The listing builds one solid part. Answer for the finished solid, in the listing's coordinates (mm). Face numbers are marked on the shaded views. Round coordinates to 2 decimals unless told otherwise and drop trailing zeros. Write each loop counter-clockwise with the first axis right and the second up, starting at its lowest first coordinate (ties: lowest second). Pieces come first, ordered by that corner, then holes. Notation, with made-up numbers: (72.25, 34.5) - (120.25, 34.5) arc R25 ccw to (120.25, 62.5) - close; hole circle Ø5 at (-18.5, 35). An arc over 180 degrees is marked (long way). Answer in a Markdown table with one row per item.
Autodesk Inventor part; units mm, degrees
ref_plane "YZ Plane" through (0, 0, 0) normal (1, 0, 0) x (0, 1, 0)
ref_plane "XZ Plane" through (0, 0, 0) normal (0, 1, 0) x (-1, 0, 0)
ref_plane "XY Plane" through (0, 0, 0) normal (0, 0, 1) x (1, 0, 0)
ref_plane "Work Plane1" through (0, 0, 2) normal (0, 0, 1) x (1, 0, 0)
sketch "Sketch1" plane through (0, 0, 2) normal (0, 0, 1) x (1, 0, 0)
  circle A0 centre (-37.0712, 14) radius 3.25 construction
  circle A1 centre (-9.0712, -14) radius 3.25 construction
  line L0 (-26.0712, -17.08) -> (-20.0712, -17.08) construction
  arc A2 (-20.0712, -17.08) -> (-20.0712, -14.08) centre (-20.0712, -15.58) ccw construction
  line L1 (-20.0712, -14.08) -> (-26.0712, -14.08) construction
  line L2 (-37.0712, -3) -> (-37.0712, 3) construction
  arc A3 (-37.0712, 3) -> (-40.0712, 3) centre (-38.5712, 3) ccw construction
  line L3 (-40.0712, 3) -> (-40.0712, -3) construction
  line L4 (-47.9712, -17) -> (-47.9712, 17) construction
  line L5 (-47.9712, 17) -> (-44.3964, 17) construction
  line L6 (-44.3964, 17) -> (-40.0712, 21.3252) construction
  line L7 (-40.0712, 21.3252) -> (-40.0712, 24.9) construction
  line L8 (-40.0712, 24.9) -> (-6.0712, 24.9) construction
  line L9 (-6.0712, 24.9) -> (-6.0712, 21.3252) construction
  line L10 (-6.0712, 21.3252) -> (-1.746, 17) construction
  line L11 (-1.746, 17) -> (1.8288, 17) construction
  line L12 (1.8288, 17) -> (1.8288, -17) construction
  line L13 (1.8288, -17) -> (-1.746, -17) construction
  line L14 (-1.746, -17) -> (-6.1126, -21.3666) construction
  line L15 (-6.1126, -21.3666) -> (-6.1126, -24.9) construction
  line L16 (-6.1126, -24.9) -> (-40.0712, -24.9) construction
  circle A4 centre (-37.0712, -14) radius 3.25 construction
  circle A5 centre (-23.0712, 0) radius 12.45 construction
  circle A6 centre (-23.0712, 0) radius 12.7 construction
  line L17 (-37.0712, 14) -> (-9.0712, 14) construction
  line L18 (-9.0712, 14) -> (-9.0712, -14) construction
  line L19 (-9.0712, -14) -> (-37.0712, -14) construction
  line L20 (-37.0712, -14) -> (-37.0712, 14) construction
  line L21 (-4.0712, -19) -> (-4.0712, 19)
  line L22 (-4.0712, 19) -> (-42.0712, 19)
  line L23 (-42.0712, 19) -> (-42.0712, -19)
  line L24 (-42.0712, -19) -> (-4.0712, -19)
  circle A7 centre (-23.0712, 0) radius 12.8
  circle A8 centre (-23.0712, 0) radius 3.25
  line L25 (-40.0712, -24.9) -> (-40.0712, -21.3252)
  line L26 (-40.0712, -21.3252) -> (-44.3964, -17)
  line L27 (-44.3964, -17) -> (-47.9712, -17)
  arc A9 (-26.0712, -14.08) -> (-26.0712, -17.08) centre (-26.0712, -15.58) ccw
  arc A10 (-40.0712, -3) -> (-37.0712, -3) centre (-38.5712, -3) ccw
  circle A11 centre (-37.0712, -14) radius 3.25
  point P0 (0, 0)
  point P1 (-21.8762, -3.0223)
  point P2 (-25.9925, 1.4242)
  dimension "d0" = 5
  dimension "d1" = 0.1
extrude "Extrusion1" add sketch "Sketch1" along normal blind 6 contours L24 L23 L22 L21 | A7 | A11
sketch "Sketch2" plane through (0, 0, 2) normal (0, 0, -1) x (-1, 0, 0)
  circle A0 centre (23.0712, 0) radius 12.8
  circle A1 centre (23.0712, 0) radius 8.5824
  point P0 (0, 0)
extrude "Extrusion2" add sketch "Sketch2" against normal blind 0.5
sketch "Sketch3" plane through (0, 0, 2) normal (0, 0, -1) x (-1, 0, 0)
  circle A0 centre (9.0712, -14) radius 1.45 construction
  circle A1 centre (9.0712, -14) radius 2.45
  circle A2 centre (37.0712, -14) radius 1.45
  circle A3 centre (37.0712, -14) radius 1.95
  point P0 (0, 0)
  dimension "d8" = 1
  dimension "d10" = 0.5
sketch "Sketch5" plane through (0, 0, 2) normal (0, 0, -1) x (-1, 0, 0)
  arc A0 (20.0712, -14.08) -> (20.0712, -17.08) centre (20.0712, -15.58) ccw
  arc A1 (26.0712, -17.08) -> (26.0712, -14.08) centre (26.0712, -15.58) ccw
  line L0 (37.0712, 3) -> (37.0712, -3)
  arc A2 (37.0712, -3) -> (40.0712, -3) centre (38.5712, -3) ccw
  line L1 (40.0712, -3) -> (40.0712, 3)
  arc A3 (40.0712, 3) -> (37.0712, 3) centre (38.5712, 3) ccw
  line L2 (26.0712, -14.08) -> (20.0712, -14.08)
  arc A4 (20.0712, -14.08) -> (20.0712, -17.08) centre (20.0712, -15.58) ccw
  line L3 (20.0712, -17.08) -> (26.0712, -17.08)
  arc A5 (26.0712, -17.08) -> (26.0712, -14.08) centre (26.0712, -15.58) ccw
  circle A6 centre (37.0712, -14) radius 1.45
  circle A7 centre (23.0712, 0) radius 1.45
  circle A8 centre (9.0712, -14) radius 1.45
  circle A9 centre (37.0712, 14) radius 1.45
  line L4 (-1.8288, -17) -> (-1.8288, 17)
  line L5 (-1.8288, 17) -> (1.746, 17)
  line L6 (1.746, 17) -> (6.0712, 21.3252)
  line L7 (6.0712, 21.3252) -> (6.0712, 24.9)
  line L8 (6.0712, 24.9) -> (40.0712, 24.9)
  line L9 (40.0712, 24.9) -> (40.0712, 21.3252)
  line L10 (40.0712, 21.3252) -> (44.3964, 17)
  line L11 (44.3964, 17) -> (47.9712, 17)
  line L12 (47.9712, 17) -> (47.9712, -17)
  line L13 (44.3964, -17) -> (47.9712, -17)
  line L14 (40.0712, -21.3252) -> (44.3964, -17)
  line L15 (40.0712, -24.9) -> (40.0712, -21.3252)
  line L16 (6.1126, -24.9) -> (40.0712, -24.9)
  line L17 (6.1126, -24.9) -> (6.1126, -21.3666)
  line L18 (6.1126, -21.3666) -> (1.746, -17)
  line L19 (1.746, -17) -> (-1.8288, -17)
  point P0 (0, 0)
  point P1 (40.0712, -3)
extrude "Extrusion5" cut sketch "Sketch5" against normal blind 8 contours L2 A1 L3 A0 | A3 L1 A2 L0
sketch "Sketch6" plane through (-42.0712, -19, 8) normal (0, -1, 0) x (1, 0, 0)
  line L0 (0, -6) -> (38, -6)
  line L1 (38, -6) -> (38, 0)
  line L2 (0, 0) -> (38, 0)
  line L3 (0, -6) -> (0, 0)
  line L4 (31.8, 0) -> (31.8, 0)
  circle A0 centre (19, -0.9548) radius 1.45
  point P0 (42.0712, -8)
  point P1 (4.5, 0)
  dimension "d34" = 2.9
extrude "Extrusion6" cut sketch "Sketch6" against normal blind 8 contours A0 L2 | L2 A0
pattern_circular "Circular Pattern1" count 2 over 90 about axis through (-23.0712, 0, 2) along (0, 0, -1) of "Extrusion6"
chamfer "Chamfer1" distance 3 angle 45 4 edges at (-42.0712, 19, 5) (-4.0712, 19, 5) (-4.0712, -19, 5) (-42.0712, -19, 5)
hole "Hole1" at (-37.0712, -14, 2) direction (0, 0, 1) diameter 4 depth 0.1 tip angle 115
sketch "Sketch4" plane through (-4.0712, -19, 2) normal (1, 0, 0) x (0, 0, -1)
  line L0 (2, 4.45) -> (6, 4.45)
  line L1 (2, 1.55) -> (6, 1.55)
  line L2 (0, 0) -> (0, 38)
  arc A0 (2, 19) -> (2, 19) centre (1.5, 4.4206) ccw
  line L3 (-1.3741, 5) -> (-0.1, 7)
  line L4 (-1.3741, 5) -> (-0.1, 3)
  line L5 (-0.1, 7) -> (0.6045, 7)
  line L6 (0.6045, 7) -> (0.6045, 3)
  line L7 (0.6045, 3) -> (-0.1, 3)
  line L8 (-0.1, 3) -> (-0.1, 7)
extrude "Extrusion4" cut sketch "Sketch4" against normal blind 8 contours L7 L8 L5 L2 | L2 L5 L6 L7 | L4 L3 L8
sketch "Sketch7" plane through (0, 0, 8) normal (0, 0, 1) x (1, 0, 0)
  circle A0 centre (-18.0712, -10.5) radius 1
  circle A1 centre (-33.5712, 11) radius 1
  circle A2 centre (-13.0712, 17.5) radius 1
  circle A3 centre (-18.0712, -10.5) radius 0.9
  circle A4 centre (-33.5712, 11) radius 0.9
  circle A5 centre (-13.0712, 17.5) radius 0.9
  point P0 (0, 0)
  dimension "d44" = 1.8
  dimension "d45" = 1.8
  dimension "d46" = 1.8
extrude "Extrusion7" cut sketch "Sketch7" against normal through all contours A3 | A4 | A5
ref_plane "Arbeitsebene2" through (-23.0712, 0, 7.0452) normal (-1, 0, 0) x (0, 0, 1)
ref_plane "Arbeitsebene3" through (-23.0712, 0, 7.0452) normal (0, -1, 0) x (1, 0, 0)
properties part number "20_Cube_Insert_Kinematic_Mirrormount_90_pro_v3"
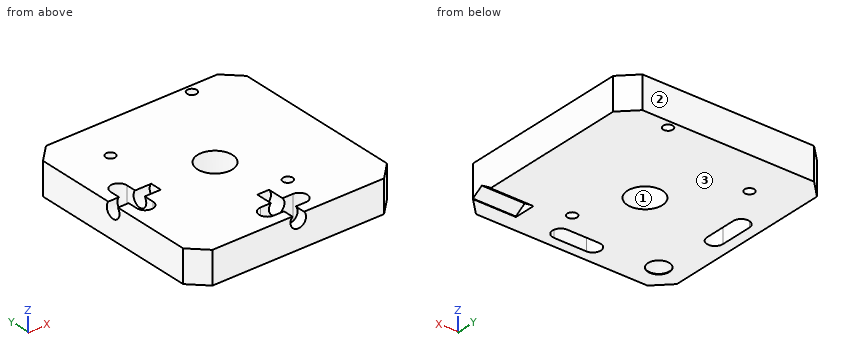
(1) Section C-C (z = 4) is taken. Give the vertices of the cut face in (x, y).
Checked values:
| item | result |
|---|---|
| outline | (-42.07, -16) - (-39.07, -19) - (-7.07, -19) - (-4.07, -16) - (-4.07, 16) - (-7.07, 19) - (-39.07, 19) - (-42.07, 16) - close; hole (-40.07, -3) arc R1.5 ccw to (-37.07, -3) - (-37.07, 3) arc R1.5 ccw to (-40.07, 3) - close; hole circle Ø1.8 at (-33.57, 11); hole circle Ø6.5 at (-23.07, 0); hole (-26.07, -17.08) - (-20.07, -17.08) arc R1.5 ccw to (-20.07, -14.08) - (-26.07, -14.08) arc R1.5 ccw to start; hole circle Ø1.8 at (-18.07, -10.5); hole circle Ø1.8 at (-13.07, 17.5) |
(2) Flat-ended cylindrical pins translate along their axes: pin 1 (2.5 mm diameter, centred on x = -18.07, y = -10.5, fed in from -Z); pin 2 (0.7 mm diameter, centred on x = -23.5, z = 6.5, fed in from -Y); pin 3 (3.5 mm diameter, centred on x = -37.07, y = -14, fed in from -Z); pin 4 (1.6 mm diameter, centred on x = -13.07, y = 17.5, fed in from -Z). Find the tip coordinate at first contact, or state that the pin passes through.
Checked values:
| item | result |
|---|---|
| pin 1 | stops at z = 2 |
| pin 2 | stops at y = -11 |
| pin 3 | stops at z = 2.26 |
| pin 4 | passes through |
(3) Section D-D (x = -13.5) is taken. Give the vertices of the cut face in (y, z).
Checked values:
| item | result |
|---|---|
| outline | (-19, 2) - (16.71, 2) - (16.71, 8) - (-19, 8) - close; (18.29, 2) - (19, 2) - (19, 8) - (18.29, 8) - close |
(4) Section A-A (y = 11) is taken. Give the vertices of the cut face in (x, z), and give its area (3 significant figures).
Checked values:
| item | result |
|---|---|
| outline | (-42.07, 2) - (-34.47, 2) - (-34.47, 8) - (-42.07, 8) - close; (-32.67, 2) - (-4.07, 2) - (-4.07, 8) - (-32.67, 8) - close |
| area | 217 mm2 |
(5) Section B-B (y = 0) is taken. Give the vertices of the cut face in (x, z), and give its area (3 significant figures).
Checked values:
| item | result |
|---|---|
| outline | (-42.07, 2) - (-40.07, 2) - (-40.07, 5.6) - (-42.07, 5.6) - close; (-37.07, 2) - (-26.32, 2) - (-26.32, 8) - (-34.07, 8) - (-34.07, 5.6) - (-37.07, 5.6) - close; (-19.82, 2) - (-4.07, 2) - (-4.07, 8) - (-19.82, 8) - close |
| area | 159 mm2 |
(6) For a pull along Y with two mould halves and no side action, classify the marked faces 1, 2 and 3 as pulls with the +Y half, pulls with the -Y half, needs draft (parallel to the pull), parting line crosses it, or undercut.
Checked values:
| item | result |
|---|---|
| face 1 | undercut |
| face 2 | pulls with the +Y half |
| face 3 | needs draft |
(7) Find the intervals of material crossed by line 1 (Y direction, x = -26, z = 3.5); line 2 (X direction, y = -3, z = 3.75); line 3 (Y direction, x = -33.5, z = 4.25), in increasing order.
Checked values:
| item | result |
|---|---|
| line 1 | y = -19 to -17.08, -14.08 to -1.41, 1.41 to 19 |
| line 2 | x = -42.07 to -40.07, -37.07 to -24.32, -21.82 to -4.07 |
| line 3 | y = -19 to 10.1, 11.9 to 19 |
